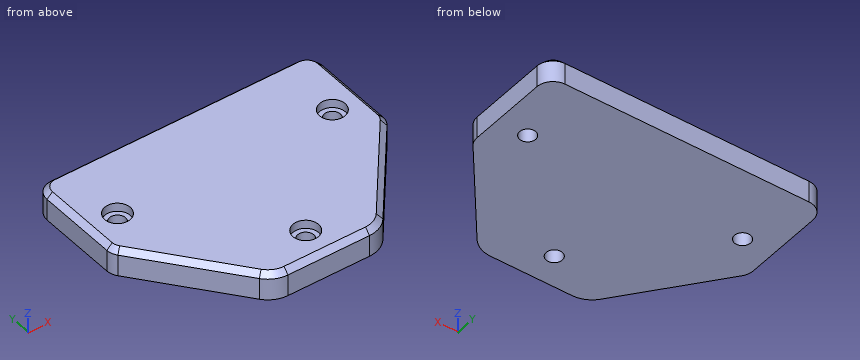
from build123d import *

# Parameters (mm, degrees)
CROQUIS1_R                   = 1.5
SALIENTE_EXTRUIR1_DEPTH      = 5
CHAFL_N1_SIZE                = 1
TALADROAVANZADO1_START       = 3.4252
TALADROAVANZADO1_OUTLINE_R   = 2.38125
TALADROAVANZADO1_OUTLINE_R_2 = 1.5
TALADROAVANZADO1_DEPTH       = 1.5748


# Read off the part's stored shape, not the designer's step: TaladroAvanzado1
with BuildPart() as part:
    # Croquis1 → Saliente-Extruir1 (new body)
    with BuildSketch(Plane.XY):
        with BuildLine():
            Line((-7.5911494, -25.7), (7.5911494, -25.7))
            ThreePointArc((7.5911494, -25.7), (9.761282919, -25.204500029), (11.501296, -23.816208204))
            Line((11.501296, -23.816208204), (25.04608796, -6.820513834))
            ThreePointArc((25.04608796, -6.820513834), (25.531807186, -5.941176745), (25.7, -4.950788912))
            Line((25.7, -4.950788912), (25.7, 9.85))
            ThreePointArc((25.7, 9.85), (24.821320344, 11.971320344), (22.7, 12.85))
            Line((22.7, 12.85), (0, 12.85))
            Line((0, 12.85), (-22.7, 12.85))
            ThreePointArc((-22.7, 12.85), (-24.821320344, 11.971320344), (-25.7, 9.85))
            Line((-25.7, 9.85), (-25.7, -4.950788912))
            ThreePointArc((-25.7, -4.950788912), (-25.531807186, -5.941176745), (-25.04608796, -6.820513834))
            Line((-25.04608796, -6.820513834), (-11.501296, -23.816208204))
            ThreePointArc((-11.501296, -23.816208204), (-9.761282919, -25.204500029), (-7.5911494, -25.7))
        make_face()
        with Locations((-20, 0)):
            Circle(CROQUIS1_R, mode=Mode.SUBTRACT)
        with Locations(Location((20, 0, 0), (0, 0, 180))):
            Circle(CROQUIS1_R, mode=Mode.SUBTRACT)
        with Locations((0, -20)):
            Circle(CROQUIS1_R, mode=Mode.SUBTRACT)
    extrude(amount=SALIENTE_EXTRUIR1_DEPTH)

    # Chaflán1
    chafl_n1_edges = [part.edges().sort_by_distance(p)[0] for p in [
        (-25.7, 2.449605544, 5),
        (-25.531807186, -5.941176745, 5),
        (-18.27369198, -15.318361019, 5),
        (-9.761282919, -25.204500029, 5),
        (0, -25.7, 5),
        (9.761282919, -25.204500029, 5),
        (18.27369198, -15.318361019, 5),
        (25.531807186, -5.941176745, 5),
        (25.7, 2.449605544, 5),
        (24.821320344, 11.971320344, 5),
        (0, 12.85, 5),
        (-24.821320344, 11.971320344, 5),
    ]]
    chamfer(chafl_n1_edges, length=CHAFL_N1_SIZE)

    # TaladroAvanzado1 outline → TaladroAvanzado1 (cut)
    # profile 1 of 3: a face of its own
    with BuildSketch(Plane.XY.offset(TALADROAVANZADO1_START)):
        with Locations((0, -20)):
            Circle(TALADROAVANZADO1_OUTLINE_R)
        with Locations((0, -20)):
            Circle(TALADROAVANZADO1_OUTLINE_R_2, mode=Mode.SUBTRACT)
    # profile 2 of 3: a face of its own
    with BuildSketch(Plane.XY.offset(TALADROAVANZADO1_START)):
        with Locations((20, 0)):
            Circle(TALADROAVANZADO1_OUTLINE_R)
        with Locations((20, 0)):
            Circle(TALADROAVANZADO1_OUTLINE_R_2, mode=Mode.SUBTRACT)
    # profile 3 of 3: a face of its own
    with BuildSketch(Plane.XY.offset(TALADROAVANZADO1_START)):
        with Locations((-20, 0)):
            Circle(TALADROAVANZADO1_OUTLINE_R)
        with Locations((-20, 0)):
            Circle(TALADROAVANZADO1_OUTLINE_R_2, mode=Mode.SUBTRACT)
    extrude(amount=TALADROAVANZADO1_DEPTH, mode=Mode.SUBTRACT)


solid = part.part
Part model, mm, in its own coordinate system. Round coordinates to 2 decimals unless told otherwise and drop trailing zeros. Write each loop counter-clockwise with the first axis right and the second up, starting at its lowest first coordinate (ties: lowest second). Pieces come first, ordered by that corner, then holes. Notation, with made-up numbers: M -13,-11 L 33,-11 A27 ccw 33,25 Z; hole C -35.75,35 d9. An arc over 180 degrees is marked long. Return JSON: item names as keys, results as strings. Group by question number.
(1) Saw through at C-C on x = 0. Write the cut outline in (y, z).
(2) Saw through at D-D on y = -20. Write the cut outline in (x, z), then the cut area to 3 significant figures.
(3) Pin check, flat tips, straight feed: pin 1 Ø2.5 at (x, y) = (0, -20) entering from -Z; pin 2 Ø12 at (x, y) = (-18.5, 2) entering from -Z; pin 3 Ø4 at (x, y) = (-20, 0) entering from +Z. Stop position of each tip, or through.
(4) Drill centre lines: probe 1 along Y at (x, z) = (0, 4.75); probe 2 along Y at (x, z) = (20, 1.55); probe 3 along Y at (x, z) = (-11.5, 2.7). Where is each one in solid material? Low to high.
(5) Saw through at A-A on z = 2.8. Write the cut outline in (x, y).
(6) Saw through at B-B on y = 0. Write the cut outline in (x, z), then the cut area to 3 significant figures.
Returned:
{
 "1": {"outline": "M -25.7,0 L -21.5,0 L -21.5,3.43 L -22.38,3.43 L -22.38,5 L -24.7,5 L -25.7,4 Z; M -18.5,0 L 12.85,0 L 12.85,4 L 11.85,5 L -17.62,5 L -17.62,3.43 L -18.5,3.43 Z"},
 "2": {"outline": "M -14.54,0 L -1.5,0 L -1.5,3.43 L -2.38,3.43 L -2.38,5 L -13.26,5 L -14.54,4 Z; M 1.5,0 L 14.54,0 L 14.54,4 L 13.26,5 L 2.38,5 L 2.38,3.43 L 1.5,3.43 Z", "area": "126 mm²"},
 "3": {"pin 1": "through", "pin 2": "z = 0", "pin 3": "z = 3.43"},
 "4": {"probe 1": "-24.95 to -22.38, -17.62 to 12.1", "probe 2": "-13.15 to -1.5, 1.5 to 12.85", "probe 3": "-23.82 to 12.85"},
 "5": {"outline": "M -25.7,-4.95 A3 ccw -25.05,-6.82 L -11.5,-23.82 A5 ccw -7.59,-25.7 L 7.59,-25.7 A5 ccw 11.5,-23.82 L 25.05,-6.82 A3 ccw 25.7,-4.95 L 25.7,9.85 A3 ccw 22.7,12.85 L -22.7,12.85 A3 ccw -25.7,9.85 Z; hole C -20,0 d3; hole C 0,-20 d3; hole C 20,0 d3"},
 "6": {"outline": "M -25.7,0 L -21.5,0 L -21.5,3.43 L -22.38,3.43 L -22.38,5 L -24.7,5 L -25.7,4 Z; M -18.5,0 L 18.5,0 L 18.5,3.43 L 17.62,3.43 L 17.62,5 L -17.62,5 L -17.62,3.43 L -18.5,3.43 Z; M 21.5,0 L 25.7,0 L 25.7,4 L 24.7,5 L 22.38,5 L 22.38,3.43 L 21.5,3.43 Z", "area": "220 mm²"}
}
